The listing builds one solid part. Answer for the finished solid, in the listing's coordinates (mm). Coordinates: 2 decimals unless noted, no trailing zeros. Write each loop counter-clockwise with the first axis right and the second up, starting at its lowest first coordinate (ties: lowest second). Pieces come first, ordered by that corner, then holes.
(1) For a pull along Y with two mould halves and no side action, classify faces 1 (the cylindrical face through (27.452, 10.112, 1.972)), 2 (the flat face through (50, 40, 2)), 3 (the flat face through (30, 24, 4)) as +Y half, -Y half, draft (parallel to the pull), parting line (faces both ways), or undercut.
(2) Straight lines are drawn through the part: line 1 (Y direction, x = 30, z = 1.35); line 2 (Y direction, x = 10, z = 1.1); line 3 (Y direction, x = 29, z = 0.3). For each, find the intervals that lie inside material, in ascending order.
(3) The part is cut by section B-B on y = 30. Determine the outline of the cut face in (x, z), plus the area to 3 significant figures.
(4) The part is cut by section A-A on x = 30. Determine the outline of the cut face in (y, z).
(5) The part is cut by section C-C on z = 3.25. Determine the outline of the cut face in (x, y), plus the area to 3 significant figures.
from build123d import *

# Parameters (mm, degrees)
SKETCH_R  = 2.55
PAD_DEPTH = 4


with BuildPart() as part:
    # Sketch → Pad (new body)
    with BuildSketch(Plane.XY):
        Polygon((0, 0), (60, 0), (60, 20), (40, 60), (20, 60), (0, 20), align=None)
        with Locations((30, 10)):
            Circle(SKETCH_R, mode=Mode.SUBTRACT)
        with Locations((10, 10)):
            Circle(SKETCH_R, mode=Mode.SUBTRACT)
        with Locations((50, 10)):
            Circle(SKETCH_R, mode=Mode.SUBTRACT)
        with Locations((30, 30)):
            Circle(SKETCH_R, mode=Mode.SUBTRACT)
        with Locations((30, 50)):
            Circle(SKETCH_R, mode=Mode.SUBTRACT)
    extrude(amount=PAD_DEPTH)


solid = part.part
Model answer:
1. face 1: undercut
1. face 2: +Y half
1. face 3: draft
2. line 1: y = 0 to 7.45, 12.55 to 27.45, 32.55 to 47.45, 52.55 to 60
2. line 2: y = 0 to 7.45, 12.55 to 40
2. line 3: y = 0 to 7.65, 12.35 to 27.65, 32.35 to 47.65, 52.35 to 60
3. outline: (5, 0) - (27.45, 0) - (27.45, 4) - (5, 4) - close; (32.55, 0) - (55, 0) - (55, 4) - (32.55, 4) - close
3. area: 180 mm2
4. outline: (0, 0) - (7.45, 0) - (7.45, 4) - (0, 4) - close; (12.55, 0) - (27.45, 0) - (27.45, 4) - (12.55, 4) - close; (32.55, 0) - (47.45, 0) - (47.45, 4) - (32.55, 4) - close; (52.55, 0) - (60, 0) - (60, 4) - (52.55, 4) - close
5. outline: (0, 0) - (60, 0) - (60, 20) - (40, 60) - (20, 60) - (0, 20) - close; hole circle Ø5.1 at (10, 10); hole circle Ø5.1 at (30, 10); hole circle Ø5.1 at (30, 30); hole circle Ø5.1 at (30, 50); hole circle Ø5.1 at (50, 10)
5. area: 2,700 mm2
